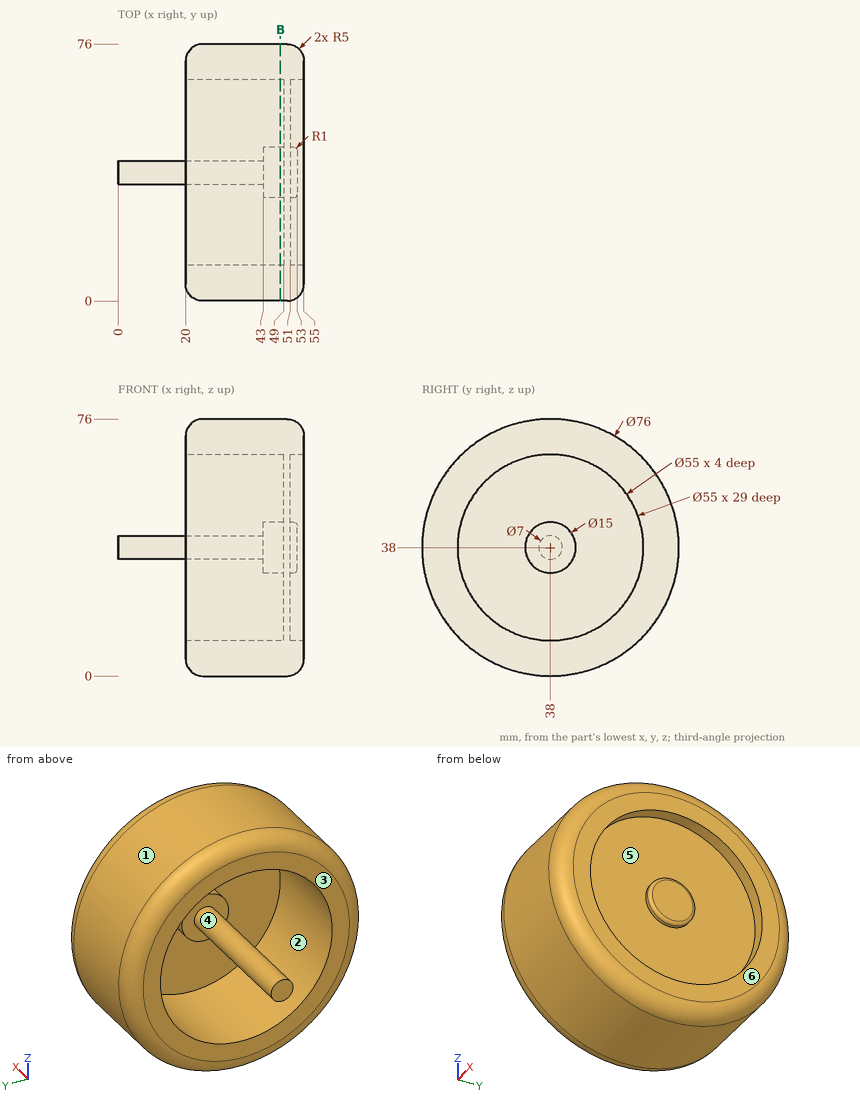
For this review, use the dimensioned drawing (mm, ordinates from the lowest corner) and the shaded views. A direction names the side the tool comes from. Coordinates: 2 decimals unless noted, no trailing zeros. Loops run counter-clockwise (first coordinate to the right, second up) from the corner with the lowest first, then second, coordinate; pieces in that order, holes last. Notation, with made-up numbers: M -35,14 L 19,14 A22 cw 19,44 Z; hole C 28.25,13.25 d8. An arc over 180 degrees is marked long. Answer as CSV lines item,"result".
Item 1: For probe 1 along Y at (x, z) = (34, 38); probe 2 along Y at (x, z) = (51.8, 38) (1 decimal); probe 3 along Z at (x, y) = (52.5, 38.5), list the stretches that pass through material, from the lowest coordinate up.
Answer list:
probe 1,"0 to 10.5, 34.5 to 41.5, 65.5 to 76"
probe 2,"0.3 to 10.5, 30.5 to 45.5, 65.5 to 75.7"
probe 3,"0.67 to 10.5, 30.65 to 45.35, 65.5 to 75.33"
Item 2: Add section B-B on x = 48. State the section outline as (y, z) points.
Answer list:
outline,"C 38,38 d76; C 38,38 d15; hole C 38,38 d55"
Item 3: For P1, Ø3, axis at x = 21, y = 12.5, coming from the +Z side; P2, Ø4, axis at x = 49.5, y = 47.5, coming from the +Z side; P3, Ø3, axis at y = 18.5, z = 39.5, coming from the +X side, all flat-tipped, find the tip position at first contact; note any pin that passes through.
Answer list:
P1,"z = 65.84"
P2,"z = 75.25"
P3,"x = 51"
Item 4: The part is to be moulded in two halves that separate along Z. For the marked faces 1, 2 and 3, say which applies: pulls with the +Z half, pulls with the -Z half, needs draft (parallel to the pull), parting line crosses it, or undercut.
Answer list:
face 1,"parting line crosses it"
face 2,"undercut"
face 3,"needs draft"
Item 5: Machinability: for the marked faces 4, 5 and 6, which of the approach directions +Z, -Z, +X, -X, +Y, -Y give a long, thin tool a straight path to every point of the face, cutting with its end or side? Answer none if there is none.
Answer list:
face 4,"-X"
face 5,"+X"
face 6,"+Z, -Z, +X, +Y, -Y"
